The model under review builds one solid part; all positions refer to its coordinate system, in mm. Round coordinates to 2 decimals unless told otherwise and drop trailing zeros. Write each loop counter-clockwise with the first axis right and the second up, starting at its lowest first coordinate (ties: lowest second). Pieces come first, ordered by that corner, then holes. Notation, with made-up numbers: M -17.5,-5.5 L 22.5,-5.5 A32 cw 22.5,26.5 Z; hole C 34,-13 d4. An arc over 180 degrees is marked long. Write item = value, one per line. Start each with the question number.
Item 1: For pin 1 Ø1.5 at (y, z) = (181.5, 22.5) entering from -X; pin 2 Ø1.5 at (y, z) = (176, -28) entering from -X; pin 3 Ø10 at (y, z) = (14.5, 7) entering from -X, all flat-tipped, find the tip position at first contact; note any pin that passes through.
Item 2: Take a section at B-B, the plane z = -22. Give the boundary of the cut face in (x, y), plus the area to 3 significant figures.
Item 3: To check wall thickness, follow line 1 along X through (y, z) = (186.5, -2); line 2 along X through (y, z) = (-218, 19); line 3 along Z through (x, y) = (15.5, 50). State the ranges of each line that lie inside material, in increasing order.
Item 4: Take a section at A-A, the plane y = -104. Give the boundary of the cut face in (x, z), plus the area to 3 significant figures.
from build123d import *

# Parameters (mm, degrees)
F1_DEPTH = 250


with BuildPart() as f1:
    # F0 (on Front) → F1 (new body, symmetric)
    with BuildSketch(Plane.XZ):
        with BuildLine():
            Line((-409.262752, -40), (0, -40))
            ThreePointArc((0, -40), (40, 0), (0, 40))
            Line((0, 40), (-409.262752, 40))
            ThreePointArc((-409.262752, 40), (-437.90667, 27.919992), (-449.24965, -1.023701))
            ThreePointArc((-449.24965, -1.023701), (-437.182744, -28.643918), (-409.262752, -40))
        make_face()
    extrude(amount=F1_DEPTH, both=True)


solid = f1.part
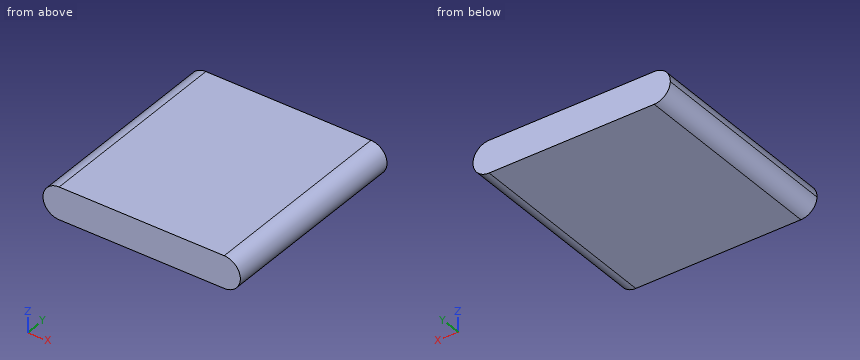
Response values:
q1.pin_1 = -442.83
q1.pin_2 = -438.54
q1.pin_3 = -449.21
q2.outline = M -442.67,-250 L 33.41,-250 L 33.41,250 L -442.67,250 Z
q2.area = 238,000 mm2
q3.line_1 = -449.21 to 39.95
q3.line_2 = -444.46 to 35.2
q3.line_3 = -36.87 to 36.87
q4.outline = M -409.26,-40 L 0,-40 A40 ccw 0,40 L -409.26,40 A40 ccw Z
q4.area = 37,800 mm2
